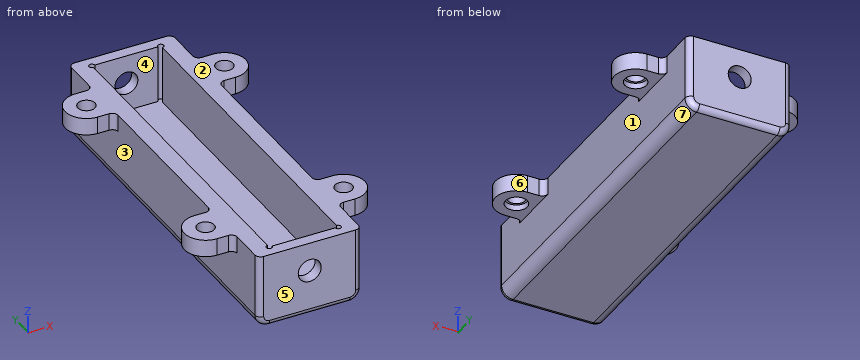
```python
from build123d import *

# Parameters (mm, degrees)
RESSALTO_EXTRUS_O1_DEPTH  = 2
ESBO_O2_R                 = 2
CORTE_EXTRUS_O1_DEPTH     = 2
RESSALTO_EXTRUS_O2_START  = -62
RESSALTO_EXTRUS_O2_DEPTH  = 62
ESBO_O4_R                 = 1.5
RESSALTO_EXTRUS_O4_DEPTH  = 3
FILETE2_R                 = 1
FILETE3_R                 = 1
ESBO_O6_R                 = 1.9
CORTE_EXTRUS_O2_DEPTH     = 1
ESPELHAR3_COPY_1_SKETCH_R = 1.5
ESPELHAR3_COPY_1_DEPTH    = 3
ESPELHAR3_COPY_2_SKETCH_R = 1.9
ESPELHAR3_COPY_2_DEPTH    = 1
FILETE4_R                 = 1
CORTE_EXTRUS_O3_START     = -10
ESBO_O7_W                 = 12
ESBO_O7_H                 = 58
CORTE_EXTRUS_O3_DEPTH     = 10
ESPELHAR5_START           = -10
ESPELHAR5_COPY_1_SKETCH_W = 12
ESPELHAR5_COPY_1_SKETCH_H = 58
ESPELHAR5_COPY_1_DEPTH    = 10


with BuildPart() as part:
    # Esboço1 → Ressalto-extrusão1 (new body)
    with BuildSketch(Plane(origin=(0, 0, 0), x_dir=(1, 0, 0), z_dir=(0, 1, 0))):
        with BuildLine():
            Line((-30.431045005, -40.729157749), (-30.431045005, -41.229157749))
            Line((-30.431045005, -41.229157749), (-29.931045005, -41.229157749))
            Line((-29.931045005, -41.229157749), (-18.931045005, -41.229157749))
            Line((-18.931045005, -41.229157749), (-18.431045005, -41.229157749))
            Line((-18.431045005, -41.229157749), (-18.431045005, -40.729157749))
            Line((-18.431045005, -40.729157749), (-18.431045005, -31.729157749))
            Line((-18.431045005, -31.729157749), (-18.431045005, -31.679157749))
            ThreePointArc((-18.431045005, -31.679157749), (-18.562846954, -31.360959697), (-18.881045005, -31.229157749))
            Line((-18.881045005, -31.229157749), (-18.931045005, -31.229157749))
            Line((-18.931045005, -31.229157749), (-29.931045005, -31.229157749))
            Line((-29.931045005, -31.229157749), (-29.981045005, -31.229157749))
            ThreePointArc((-29.981045005, -31.229157749), (-30.299243057, -31.360959697), (-30.431045005, -31.679157749))
            Line((-30.431045005, -31.679157749), (-30.431045005, -31.729157749))
            Line((-30.431045005, -31.729157749), (-30.431045005, -40.729157749))
        make_face()
    ressalto_extrus_o1 = extrude(amount=RESSALTO_EXTRUS_O1_DEPTH)

    # Esboço2 → Corte-extrusão1 (cut)
    with BuildSketch(Plane(origin=(0, 2, 0), x_dir=(1, 0, 0), z_dir=(0, 1, 0))):
        with Locations(Location((-24.431045005, -36.229157749, 0), (0, 0, 270))):
            Circle(ESBO_O2_R)
    corte_extrus_o1 = extrude(amount=-CORTE_EXTRUS_O1_DEPTH, mode=Mode.SUBTRACT)

    # Esboço3 → Ressalto-extrusão2 (add)
    with BuildSketch(Plane(origin=(0, 2, 0), x_dir=(1, 0, 0), z_dir=(0, 1, 0)).offset(RESSALTO_EXTRUS_O2_START)):
        with BuildLine():
            Line((-29.931045005, -31.229157749), (-29.981045005, -31.229157749))
            ThreePointArc((-29.981045005, -31.229157749), (-30.299243057, -31.360959697), (-30.431045005, -31.679157749))
            Line((-30.431045005, -31.679157749), (-30.431045005, -32.172163455))
            Line((-30.431045005, -32.172163455), (-30.431045005, -41.229157749))
            Line((-30.431045005, -41.229157749), (-33.431045005, -41.229157749))
            Line((-33.431045005, -41.229157749), (-33.431045005, -30.229157749))
            ThreePointArc((-33.431045005, -30.229157749), (-32.845258568, -28.814944187), (-31.431045005, -28.229157749))
            Line((-31.431045005, -28.229157749), (-17.431045005, -28.229157749))
            ThreePointArc((-17.431045005, -28.229157749), (-16.016831443, -28.814944187), (-15.431045005, -30.229157749))
            Line((-15.431045005, -30.229157749), (-15.431045005, -41.229157749))
            Line((-15.431045005, -41.229157749), (-18.431045005, -41.229157749))
            Line((-18.431045005, -41.229157749), (-18.431045005, -31.679157749))
            ThreePointArc((-18.431045005, -31.679157749), (-18.562846954, -31.360959697), (-18.881045005, -31.229157749))
            Line((-18.881045005, -31.229157749), (-29.931045005, -31.229157749))
        make_face()
    extrude(amount=RESSALTO_EXTRUS_O2_DEPTH)

    # Esboço4 → Ressalto-extrusão4 (add)
    with BuildSketch(Plane.XY.offset(41.229157749)):
        with BuildLine():
            Line((-33.431045005, -5.8), (-36.431045005, -5.8))
            ThreePointArc((-36.431045005, -5.8), (-40.131045005, -9.5), (-36.431045005, -13.2))
            Line((-36.431045005, -13.2), (-33.431045005, -13.2))
            Line((-33.431045005, -13.2), (-33.431045005, -5.8))
        make_face()
        with Locations((-36.431045005, -9.5)):
            Circle(ESBO_O4_R, mode=Mode.SUBTRACT)
    ressalto_extrus_o4 = extrude(amount=-RESSALTO_EXTRUS_O4_DEPTH)

    # Filete2
    filete2_edges = [part.edges().sort_by_distance(p)[0] for p in [
        (-33.431045005, -5.8, 39.729157749),
        (-33.431045005, -13.2, 39.729157749),
    ]]
    fillet(filete2_edges, radius=FILETE2_R)

    # Espelhar1: Ressalto-extrusão1, Corte-extrusão1 across plane
    add(ressalto_extrus_o1.mirror(Plane.ZX.offset(-29)))
    add(corte_extrus_o1.mirror(Plane.ZX.offset(-29)), mode=Mode.SUBTRACT)

    # Filete3
    filete3_edges = [part.edges().sort_by_distance(p)[0] for p in [
        (-33.431045005, -60, 35.729157749),
        (-32.845258568, -60, 28.814944187),
        (-24.431045005, -60, 28.229157749),
        (-16.016831443, -60, 28.814944187),
        (-15.431045005, -60, 35.729157749),
        (-15.431045005, 2, 35.729157749),
        (-16.016831443, 2, 28.814944187),
        (-24.431045005, 2, 28.229157749),
        (-32.845258568, 2, 28.814944187),
        (-33.431045005, 2, 35.729157749),
    ]]
    fillet(filete3_edges, radius=FILETE3_R)

    # Esboço6 → Corte-extrusão2 (cut)
    with BuildSketch(Plane(origin=(0, 0, 38.229157749), x_dir=(-1, 0, 0), z_dir=(0, 0, -1))):
        with Locations((36.431045005, -9.5)):
            Circle(ESBO_O6_R)
    corte_extrus_o2 = extrude(amount=-CORTE_EXTRUS_O2_DEPTH, mode=Mode.SUBTRACT)

    # Espelhar2: Ressalto-extrusão4, Corte-extrusão2 across plane
    add(ressalto_extrus_o4.mirror(Plane(origin=(-24.431045005, 0, 0), x_dir=(0, 0, 1), z_dir=(1, 0, 0))))
    add(corte_extrus_o2.mirror(Plane(origin=(-24.431045005, 0, 0), x_dir=(0, 0, 1), z_dir=(1, 0, 0))), mode=Mode.SUBTRACT)

    # Espelhar3: Ressalto-extrusão4, Corte-extrusão2 across plane
    add(ressalto_extrus_o4.mirror(Plane.ZX.offset(-29)))
    add(corte_extrus_o2.mirror(Plane.ZX.offset(-29)), mode=Mode.SUBTRACT)

    # Espelhar3 copy 1 sketch → Espelhar3 copy 1 (add)
    with BuildSketch(Plane(origin=(-48.86209001, -58, 41.229157749), x_dir=(-1, 0, 0), z_dir=(0, 0, 1))):
        with BuildLine():
            Line((-33.431045005, -5.8), (-36.431045005, -5.8))
            ThreePointArc((-36.431045005, -5.8), (-40.131045005, -9.5), (-36.431045005, -13.2))
            Line((-36.431045005, -13.2), (-33.431045005, -13.2))
            Line((-33.431045005, -13.2), (-33.431045005, -5.8))
        make_face()
        with Locations((-36.431045005, -9.5)):
            Circle(ESPELHAR3_COPY_1_SKETCH_R, mode=Mode.SUBTRACT)
    extrude(amount=-ESPELHAR3_COPY_1_DEPTH)

    # Espelhar3 copy 2 sketch → Espelhar3 copy 2 (cut)
    with BuildSketch(Plane(origin=(-48.86209001, -58, 38.229157749), x_dir=(1, 0, 0), z_dir=(0, 0, -1))):
        with Locations((36.431045005, -9.5)):
            Circle(ESPELHAR3_COPY_2_SKETCH_R)
    extrude(amount=-ESPELHAR3_COPY_2_DEPTH, mode=Mode.SUBTRACT)

    # Filete4
    filete4_edges = [part.edges().sort_by_distance(p)[0] for p in [
        (-15.431045005, -5.8, 39.729157749),
        (-15.431045005, -13.2, 39.729157749),
        (-15.431045005, -52.2, 39.729157749),
        (-15.431045005, -44.8, 39.729157749),
        (-33.431045005, -52.2, 39.729157749),
        (-33.431045005, -44.8, 39.729157749),
    ]]
    fillet(filete4_edges, radius=FILETE4_R)

    # Esboço7 → Corte-extrusão3 (cut)
    with BuildSketch(Plane.XY.offset(41.229157749).offset(CORTE_EXTRUS_O3_START)):
        with Locations((-24.431045005, -29)):
            Rectangle(ESBO_O7_W, ESBO_O7_H)
        with BuildLine():
            Line((-30.431045005, -0.5), (-30.431045005, 0))
            Line((-30.431045005, 0), (-29.931045005, 0))
            ThreePointArc((-29.931045005, 0), (-30.784598396, 0.353553391), (-30.431045005, -0.5))
        make_face()
    corte_extrus_o3 = extrude(amount=CORTE_EXTRUS_O3_DEPTH, mode=Mode.SUBTRACT)

    # Espelhar4: Corte-extrusão3 across plane
    add(corte_extrus_o3.mirror(Plane(origin=(-24.431045005, 0, 0), x_dir=(0, 0, 1), z_dir=(1, 0, 0))), mode=Mode.SUBTRACT)

    # Espelhar5: Corte-extrusão3 across plane
    add(corte_extrus_o3.mirror(Plane.ZX.offset(-29)), mode=Mode.SUBTRACT)

    # Espelhar5 copy 1 sketch → Espelhar5 copy 1 (cut)
    with BuildSketch(Plane(origin=(-48.86209001, -58, 41.229157749), x_dir=(-1, 0, 0), z_dir=(0, 0, 1)).offset(ESPELHAR5_START)):
        with Locations((-24.431045005, -29)):
            Rectangle(ESPELHAR5_COPY_1_SKETCH_W, ESPELHAR5_COPY_1_SKETCH_H)
        with BuildLine():
            Line((-30.431045005, -0.5), (-30.431045005, 0))
            Line((-30.431045005, 0), (-29.931045005, 0))
            ThreePointArc((-29.931045005, 0), (-30.784598396, 0.353553391), (-30.431045005, -0.5))
        make_face()
    extrude(amount=ESPELHAR5_COPY_1_DEPTH, mode=Mode.SUBTRACT)


solid = part.part
```
Source: CAD feature listing. Evaluate the final solid. Frame: model axes, mm. Face numbers are marked on the shaded views. A direction names the side the tool comes from. Coordinates: 2 decimals unless noted, no trailing zeros. Loops run counter-clockwise (first coordinate to the right, second up) from the corner with the lowest first, then second, coordinate; pieces in that order, holes last. Notation, with made-up numbers: M -23,13.25 L -18,13.25 A6 ccw -18,17.25 Z; hole C 55.25,89 d10. An arc over 180 degrees is marked long. Put each result on its own line as item: value. Start each with the question number.
1) Cut plane B-B on x = -27.5. Return the cut outline in (y, z), then the cut area to 3 significant figures.
2) Ray query, L1, parallel to X at y = -48.5, z = 40.45; L2, parallel to Y at x = -27, z = 36.25; L3, parallel to X at y = -24, z = 37.5. Return the intervals inside material, ascending. Write a range as from..to.
3) Reachability of the marked faces 1, 2, 3 and 4 from +Z, -Z, +X, -X, +Y, -Y: full face, straight path, thin tool, end or side. Return the list, or none.
4) Cut plane C-C on z = 37. Return the cut outline in (x, y), then the cut area to 3 significant figures.
5) Cut plane D-D on x = -13. Return the cut outline in (y, z).
6) Cut plane A-A on y = -48.5. Give the number of separate pieces and of enclosed holes in the cut face, then the cut area to 3 significant figures.
7) Contact query for flat-ended pins moving along their axis: pin 1 Ø1 at (x, z) = (-35.5, 40.5) entering from +Y; pin 2 Ø2 at (x, z) = (-36, 39.5) entering from -Y; pin 3 Ø10 at (x, y) = (-25, -11.5) entering from +Z. Output: stop coordinate, or through.
8) Pull-direction query (Y, two-part tool) for the marked faces 5, 6 and 7; classes: pulls with the +Y half, pulls with the -Y half, needs draft (parallel to the pull), parting line crosses it, or undercut.
The answers:
1. outline: M -60,29.23 A1 ccw -59,28.23 L 1,28.23 A1 ccw 2,29.23 L 2,41.23 L 0,41.23 L 0,31.23 L -58,31.23 L -58,41.23 L -60,41.23 Z
1. area: 226 mm²
2. L1: x = -40.13..-37.93, -34.93..-30.43, -18.43..-13.93, -10.93..-8.73
2. L2: y = -60..-58, 0..2
2. L3: x = -33.43..-30.43, -18.43..-15.43
3. face 1: -Z, +X
3. face 2: +Z, +X, -X, +Y, -Y
3. face 3: -Z, -X
3. face 4: +Z
4. outline: M -33.43,-59 A1 ccw -32.43,-60 L -26.28,-60 L -26.28,-58 L -29.93,-58 A0.5 cw long -30.43,-57.5 L -30.43,-0.5 A0.5 cw long -29.93,0 L -26.28,0 L -26.28,2 L -32.43,2 A1 ccw -33.43,1 Z; M -22.59,-60 L -16.43,-60 A1 ccw -15.43,-59 L -15.43,1 A1 ccw -16.43,2 L -22.59,2 L -22.59,0 L -18.93,0 A0.5 cw long -18.43,-0.5 L -18.43,-57.5 A0.5 cw long -18.93,-58 L -22.59,-58 Z
4. area: 402 mm²
5. outline: M -52.2,38.23 L -50.31,38.23 L -50.31,39.23 L -49.89,39.23 L -49.89,41.23 L -52.2,41.23 Z; M -47.11,39.23 L -46.69,39.23 L -46.69,38.23 L -44.8,38.23 L -44.8,41.23 L -47.11,41.23 Z; M -13.2,38.23 L -11.31,38.23 L -11.31,39.23 L -10.89,39.23 L -10.89,41.23 L -13.2,41.23 Z; M -8.11,39.23 L -7.69,39.23 L -7.69,38.23 L -5.8,38.23 L -5.8,41.23 L -8.11,41.23 Z
6. separate pieces: 3
6. enclosed holes: 0
6. area: 133 mm²
7. pin 1: stops at y = -5.8
7. pin 2: stops at y = -52.2
7. pin 3: stops at z = 31.23
8. face 5: pulls with the -Y half
8. face 6: undercut
8. face 7: needs draft
